Work out the finished part from the listing and answer in its coordinate system (mm). A direction names the side the tool comes from. Round coordinates to 2 decimals unless told otherwise and drop trailing zeros. Loops run counter-clockwise (first coordinate to the right, second up) from the corner with the lowest first, then second, coordinate; pieces in that order, holes last. Notation, with made-up numbers: (-27.5, 7.5) - (3.5, 7.5) arc R15 cw to (3.5, 34.5) - close; hole circle Ø4 at (56, 17). An arc over 180 degrees is marked (long way). Return JSON: item names as keys, results as strings.
from build123d import *

# Parameters (mm, degrees)
F1_R     = 24.5
F1_R_2   = 15.5
F1_R_3   = 2.2
F2_DEPTH = 15
F3_START = 1
F3_DEPTH = 24
F4_START = 1
F4_DEPTH = 13
F5_W     = 18
F5_H     = 13
F6_DEPTH = 24.5


with BuildPart() as f2:
    # F1 (on Top) → F2 (new body)
    with BuildSketch(Plane.XY):
        with BuildLine():
            ThreePointArc((5.5, -24.899799196), (19.8808953521, -15.9687194227), (25.5, 0))
            ThreePointArc((25.5, 0), (24.3688816797, 7.5104996957), (21.0758740643, 14.3547041914))
            ThreePointArc((21.0758740643, 14.3547041914), (20.1955865128, 15.5688241496), (19.2454493009, 16.7290968438))
            ThreePointArc((19.2454493009, 16.7290968438), (19.1021469265, 16.8809670513), (18.9690541914, 17.0418597308))
            ThreePointArc((18.9690541914, 17.0418597308), (17.9344457512, 18.1274834325), (16.8378081669, 19.1504103385))
            ThreePointArc((16.8378081669, 19.1504103385), (8.9976257046, 23.85985607), (1.63e-08, 25.5))
            ThreePointArc((1.63e-08, 25.5), (-18.0312229145, 18.031222926), (-25.5, 0))
            ThreePointArc((-25.5, 0), (-24.3688816797, -7.5104996957), (-21.0758740643, -14.3547041914))
            ThreePointArc((-21.0758740643, -14.3547041914), (-20.1955865128, -15.5688241496), (-19.2454493009, -16.7290968438))
            ThreePointArc((-19.2454493009, -16.7290968438), (-19.1021469265, -16.8809670513), (-18.9690541914, -17.0418597308))
            ThreePointArc((-18.9690541914, -17.0418597308), (-17.9344457512, -18.1274834325), (-16.8378081669, -19.1504103385))
            ThreePointArc((-16.8378081669, -19.1504103385), (-8.99762568, -23.8598560793), (3.64e-08, -25.5))
            ThreePointArc((3.64e-08, -25.5), (2.766326147, -25.3495057082), (5.5, -24.899799196))
        make_face()
        Circle(F1_R, mode=Mode.SUBTRACT)
        Circle(F1_R)
        with Locations((-1.5, -1)):
            Circle(F1_R_2, mode=Mode.SUBTRACT)
        with Locations((-1.5, -1)):
            Circle(F1_R_2)
        with BuildLine():
            Line((5.5, -25.5), (25.5, -25.5))
            Line((25.5, -25.5), (25.5, 0))
            ThreePointArc((25.5, 0), (19.8808953521, -15.9687194227), (5.5, -24.899799196))
            Line((5.5, -24.899799196), (5.5, -25.5))
        make_face()
        with BuildLine():
            ThreePointArc((-18.3, -19), (-18.4718795774, -17.9653567251), (-18.9690541914, -17.0418597308))
            ThreePointArc((-18.9690541914, -17.0418597308), (-19.1078916798, -16.88604381), (-19.2454493009, -16.7290968438))
            ThreePointArc((-19.2454493009, -16.7290968438), (-21.4071542379, -15.801347211), (-23.6190329487, -16.6021469265))
            ThreePointArc((-23.6190329487, -16.6021469265), (-23.8978530735, -21.1190329487), (-19.3809670513, -21.3978530735))
            ThreePointArc((-19.3809670513, -21.3978530735), (-18.582731977, -20.315122535), (-18.3, -19))
        make_face()
        with Locations((-21.5, -19)):
            Circle(F1_R_3, mode=Mode.SUBTRACT)
        with BuildLine():
            ThreePointArc((18.9690541914, 17.0418597308), (19.1078916798, 16.88604381), (19.2454493009, 16.7290968438))
            ThreePointArc((19.2454493009, 16.7290968438), (21.4071542379, 15.801347211), (23.6190329487, 16.6021469265))
            ThreePointArc((23.6190329487, 16.6021469265), (24.417268023, 17.684877465), (24.7, 19))
            ThreePointArc((24.7, 19), (22.815122535, 21.917268023), (19.3809670513, 21.3978530735))
            ThreePointArc((19.3809670513, 21.3978530735), (18.3142120109, 19.3012555205), (18.9690541914, 17.0418597308))
        make_face()
        with Locations((21.5, 19)):
            Circle(F1_R_3, mode=Mode.SUBTRACT)
        with BuildLine():
            Line((-19.3809670513, -21.3978530735), (-16.8378081669, -19.1504103385))
            ThreePointArc((-16.8378081669, -19.1504103385), (-17.9344457512, -18.1274834325), (-18.9690541914, -17.0418597308))
            ThreePointArc((-18.9690541914, -17.0418597308), (-18.4718795774, -17.9653567251), (-18.3, -19))
            ThreePointArc((-18.3, -19), (-18.582731977, -20.315122535), (-19.3809670513, -21.3978530735))
        make_face()
        with BuildLine():
            ThreePointArc((-19.2454493009, -16.7290968438), (-20.1955865128, -15.5688241496), (-21.0758740643, -14.3547041914))
            Line((-21.0758740643, -14.3547041914), (-23.6190329487, -16.6021469265))
            ThreePointArc((-23.6190329487, -16.6021469265), (-21.4071542379, -15.801347211), (-19.2454493009, -16.7290968438))
        make_face()
        with BuildLine():
            ThreePointArc((19.2454493009, 16.7290968438), (20.1955865128, 15.5688241496), (21.0758740643, 14.3547041914))
            Line((21.0758740643, 14.3547041914), (23.6190329487, 16.6021469265))
            ThreePointArc((23.6190329487, 16.6021469265), (21.4071542379, 15.801347211), (19.2454493009, 16.7290968438))
        make_face()
        with BuildLine():
            Line((19.3809670513, 21.3978530735), (16.8378081669, 19.1504103385))
            ThreePointArc((16.8378081669, 19.1504103385), (17.9344457512, 18.1274834325), (18.9690541914, 17.0418597308))
            ThreePointArc((18.9690541914, 17.0418597308), (18.3142120109, 19.3012555205), (19.3809670513, 21.3978530735))
        make_face()
        with BuildLine():
            ThreePointArc((-19.2454493009, -16.7290968438), (-19.1078916798, -16.88604381), (-18.9690541914, -17.0418597308))
            ThreePointArc((-18.9690541914, -17.0418597308), (-19.1021469265, -16.8809670513), (-19.2454493009, -16.7290968438))
        make_face()
        with BuildLine():
            ThreePointArc((18.9690541914, 17.0418597308), (19.1021469265, 16.8809670513), (19.2454493009, 16.7290968438))
            ThreePointArc((19.2454493009, 16.7290968438), (19.1078916798, 16.88604381), (18.9690541914, 17.0418597308))
        make_face()
    extrude(amount=F2_DEPTH)

    # F1 (on Top) → F3 (cut)
    with BuildSketch(Plane.XY.offset(F3_START)):
        with Locations((-1.5, -1)):
            Circle(F1_R_2)
    extrude(amount=F3_DEPTH, mode=Mode.SUBTRACT)

    # F1 (on Top) → F4 (cut)
    with BuildSketch(Plane.XY.offset(F4_START)):
        Circle(F1_R)
        with Locations((-1.5, -1)):
            Circle(F1_R_2, mode=Mode.SUBTRACT)
        with Locations((-1.5, -1)):
            Circle(F1_R_2)
    extrude(amount=F4_DEPTH, mode=Mode.SUBTRACT)

    # F5 (on face) → F6 (cut, through all)
    with BuildSketch(Plane.XZ.offset(25.5)):
        with Locations((15.5, 7.5)):
            Rectangle(F5_W, F5_H)
    extrude(amount=-F6_DEPTH, mode=Mode.SUBTRACT)


solid = f2.part
1) Find the intervals of material crossed by L1, parallel to Z at x = 13, y = -15.5; L2, parallel to X at y = 20.5, z = 10; L3, parallel to Z at x = -14.5, y = -1, in increasing order.
Verdict:
{"L1": "z = 0 to 1, 14 to 15", "L2": "x = -15.17 to -13.42, 13.42 to 15.17, 18.36 to 19.89, 23.11 to 24.33", "L3": "z = 0 to 1"}
2) A tool of negligible diameter and unlimited length cuts with its end or side. For faces 4 (the flat face through (18.13, 20.29, 7.4)), 5 (the cylindrical face through (-18.63, 15.91, 7.41)), 6 (the flat face through (24.5, -13, 7)), from which of +Z, -Z, +X, -X, +Y, -Y can it reach the whole face along a straight path? Write none if from no direction.
Verdict:
{"face 4": "+Z, -Z, +Y", "face 5": "none", "face 6": "-Y"}
3) Section C-C (y = -10) is taken. Give the vertices of the cut face in (x, z), and give its area (3 significant figures).
Verdict:
{"outline": "(-23.46, 0) - (25.5, 0) - (25.5, 15) - (11.12, 15) - (11.12, 14) - (24.5, 14) - (24.5, 1) - (-22.37, 1) - (-22.37, 14) - (-14.12, 14) - (-14.12, 15) - (-23.46, 15) - close", "area": "99.9 mm2"}
4) Section B-B (x = 10) is taken. Give the vertices of the cut face in (y, z), and give its area (3 significant figures).
Verdict:
{"outline": "(-25.5, 0) - (23.46, 0) - (23.46, 15) - (9.39, 15) - (9.39, 14) - (22.37, 14) - (22.37, 1) - (-25.5, 1) - close; (-25.5, 14) - (-11.39, 14) - (-11.39, 15) - (-25.5, 15) - close", "area": "91.3 mm2"}
5) Flat-ended cylindrical pins translate along their axes: pin 1 (1.5 mm diameter, centred on x = 19.5, z = 2, fed in from +Y); pin 2 (3 mm diameter, centred on y = 5, z = 2.5, fed in from +X); pin 3 (4 mm diameter, centred on y = -14, z = 6.5, fed in from -X). Find the tip coordinate at first contact, or state that the pin passes through.
Verdict:
{"pin 1": "stops at y = 21.95", "pin 2": "stops at x = 25.26", "pin 3": "stops at x = -22.94"}
6) Determine the mould class of faces 1 (the flat face through (-22.33, -15.463, 7.395)), 2 (the flat face through (0, -1, 1)), 3 (the cylindrical face through (24.4, 7.41, 7.4)) for opening direction X: pulls with the +X half, pulls with the -X half, needs draft (parallel to the pull), parting line crosses it, or undercut.
Verdict:
{"face 1": "pulls with the -X half", "face 2": "undercut", "face 3": "pulls with the +X half"}
7) Section A-A (z = 5.25) is taken. Count the separate pieces of the cut face and the enclosed holes in it, and give its area (3 significant figures).
Verdict:
{"separate pieces": "1", "enclosed holes": "2", "area": "194 mm2"}
8) Section D-D (x = -9.5) is taken. Give the vertices of the cut face in (y, z).
Verdict:
{"outline": "(-23.66, 0) - (23.66, 0) - (23.66, 15) - (12.28, 15) - (12.28, 14) - (22.58, 14) - (22.58, 1) - (-22.58, 1) - (-22.58, 14) - (-14.28, 14) - (-14.28, 15) - (-23.66, 15) - close"}
